The listing builds one solid part. Answer for the finished solid, in the listing's coordinates (mm). Face numbers are marked on the shaded views. Give positions to 0.01 mm unless a question says otherwise; leave off trailing zeros. Write each loop counter-clockwise with the first axis right and the second up, starting at its lowest first coordinate (ties: lowest second). Pieces come first, ordered by that corner, then holes. Notation, with made-up numbers: (65.5, 31.5) -> (113.5, 31.5) arc R25 ccw to (113.5, 47.5) -> close; hole circle Ø11 at (-26.75, 85). An arc over 180 degrees is marked (long way). Put each result on its own line as item: value. Start each with the question number.
1) Find the intervals of material crossed by line 1 along Y through (x, z) = (-8.5, -9); line 2 along Y through (x, z) = (5, -13.5); line 3 along X through (y, z) = (-17, -38), in increasing order. Write a range as from..to.
2) A cutting plane is placed at C-C (x = 25.5). Write down the section's boundary in (y, z).
3) A cutting plane is placed at A-A (z = 11.5). Write down the section's boundary in (x, y), then the cut area to 3 significant figures.
4) For a pull along Y with two mould halves and no side action, classify the marked faces 1, 2 and 3 as released by +Y, released by -Y, zero draft, split by the parting line, or undercut.
5) Flat-ended cylindrical pins translate along their axes: pin 1 Ø5 at (y, z) = (-9.5, -13) entering from +X; pin 2 Ø4.5 at (x, y) = (-17.6, -0.09) entering from +Z; pin 3 Ø6 at (y, z) = (-35.5, 37.5) entering from +X. Find the tip coordinate at first contact, or state that the pin passes through.
6) A cutting plane is placed at B-B (y = -54). Write down the section's boundary in (x, z), then the cut area to 3 significant figures.
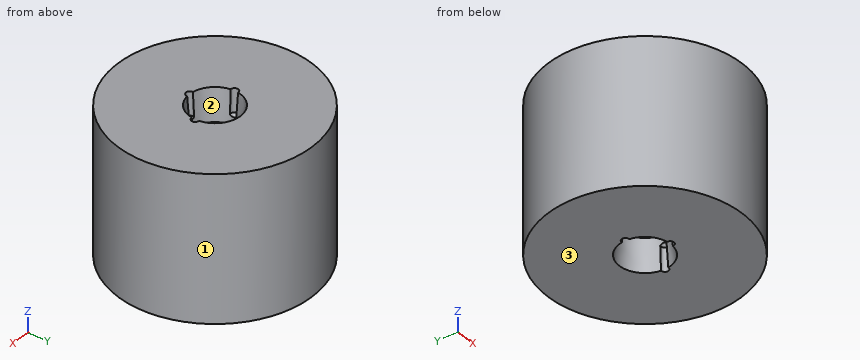
Autodesk Inventor part; units mm, degrees
ref_plane "YZ Plane" through (0, 0, 0) normal (1, 0, 0) x (0, 1, 0)
ref_plane "XZ Plane" through (0, 0, 0) normal (0, 1, 0) x (-1, 0, 0)
ref_plane "XY Plane" through (0, 0, 0) normal (0, 0, 1) x (1, 0, 0)
sketch "Esquisse3" plane through (0, 0, 0) normal (1, 0, 0) x (0, 1, 0)
  line L0 (12.5, 50) -> (17.6, 50)
  line L1 (12.5, 27.7) -> (16, 27.7)
  line L2 (16, 27.7) -> (17.6, 50)
  line L3 (-39.3437, 0) -> (46.6159, 0)
  line L4 (12.5, -50) -> (17.6, -50)
  line L5 (12.5, -27.7) -> (16, -27.7)
  line L6 (16, -27.7) -> (17.6, -50)
  line L7 (12.5, -50) -> (12.5, -27.7)
  line L8 (0, 98.6871) -> (0, -122.4022)
  line L9 (17.6, 50) -> (67, 50)
  line L10 (67, 50) -> (67, -50)
  line L11 (67, -50) -> (17.6, -50)
  line L12 (12.5, 50) -> (12.5, 27.7)
  line L13 (12.5, 27.7) -> (12.5, -27.7)
  point P0 (0, 0)
  point P1 (40.7356, 59.8426)
  point P2 (56.7464, 59.8426)
  point P3 (58.3249, 81.8426)
  point P4 (40.7356, 81.8426)
  dimension "d14" = 22.3
  dimension "d19" = 0
  dimension "d20" = 100
  dimension "d21" = 0
  dimension "d22" = 25
  dimension "d23" = 134
  dimension "d25" = 35.2
  dimension "d26" = 32
revolve "Révolution1" add sketch "Esquisse3" angle 360 about axis through (0, 0, 98.6871) along (0, 0, -1) contours L9 L10 L11 L6 L5 L13 L1 L2
sketch "Esquisse4" plane through (0, 0, 50) normal (0, 0, 1) x (1, 0, 0)
  circle A0 centre (0, 0) radius 17.6
  line L0 (-27.4685, -0.0852) -> (22.7682, -0.0852)
  line L1 (0, 22.4796) -> (0, -21.2618)
  point P0 (0, 0)
  point P1 (17.5998, -0.0852)
  point P2 (0, -17.6)
  point P3 (-17.5998, -0.0852)
hole "Perçage2" at (17.5998, -0.0852, 50) at (0, -17.6, 50) at (-17.5998, -0.0852, 50) direction (0, 0, -1) diameter 5.134 depth 16.2 tip angle 118
mirror "Mise en miroir1" about plane through (0, 0, 0) normal (0, 0, 1) of "Perçage2"
properties part number "Masse"
Reply:
1. line 1: y = -66.46..-9.17, 9.17..66.46
1. line 2: y = -66.81..-11.46, 11.46..66.81
1. line 3: x = -64.81..-2.5, 2.5..64.81
2. outline: (-61.96, -50) -> (61.96, -50) -> (61.96, 50) -> (-61.96, 50) -> close
3. outline: circle Ø134 at (0, 0); hole circle Ø25 at (0, 0)
3. area: 13,600 mm2
4. face 1: split by the parting line
4. face 2: undercut
4. face 3: zero draft
5. pin 1: stops at x = 66.63
5. pin 2: stops at z = 33.61
5. pin 3: stops at x = 58.59
6. outline: (-39.66, -50) -> (39.66, -50) -> (39.66, 50) -> (-39.66, 50) -> close
6. area: 7,930 mm2
